The model under review builds one solid part; all positions refer to its coordinate system, in mm. A direction names the side the tool comes from. Coordinates: 2 decimals unless noted, no trailing zeros. Write each loop counter-clockwise with the first axis right and the second up, starting at its lowest first coordinate (ties: lowest second). Pieces come first, ordered by that corner, then holes.
```python
from build123d import *

# Parameters (mm, degrees)
SCHIZZO1_R                                   = 40
ESTRUSIONE_ESTRUSIONE1_DEPTH                 = 45
SCHIZZO2_W                                   = 156
SCHIZZO2_H                                   = 140
SCHIZZO2_R                                   = 30
ESTRUSIONE_ESTRUSIONE2_DEPTH                 = 25
ESTRUSIONE_ESTRUSIONE4_DEPTH                 = 10
SCHIZZO6_R                                   = 12.5
TAGLIO_ESTRUSIONE1_DEPTH                     = 10
FORO_LAMATO_PER_VITE_M4_A_TESTA_ESAG_2_COUNT = 2
FORO_LAMATO_PER_VITE_M4_A_TESTA_ESAG_2_PITCH = 36.062445841
FORO_LAMATO_PER_VITE_M4_A_TESTA_ESAG_3_COUNT = 2
FORO_LAMATO_PER_VITE_M4_A_TESTA_ESAG_3_PITCH = 51
FORO_LAMATO_PER_VITE_M4_A_TESTA_ESAG_4_COUNT = 2
FORO_LAMATO_PER_VITE_M4_A_TESTA_ESAG_4_PITCH = 36.062445841
FORO_PER_VITE_M5_1_D                         = 5.5


with BuildPart() as part:
    # Schizzo1 → Estrusione-Estrusione1 (new body)
    with BuildSketch(Plane(origin=(0, 0, 0), x_dir=(0, 0, -1), z_dir=(1, 0, 0))):
        with BuildLine():
            Line((-70, 0), (-70, 136.8))
            Line((-70, 136.8), (70, 136.8))
            Line((70, 136.8), (70, 0))
            ThreePointArc((70, 0), (0, -70), (-70, 0))
        make_face()
        with Locations(Location((0, 0, 0), (0, 0, 180))):
            Circle(SCHIZZO1_R, mode=Mode.SUBTRACT)
    extrude(amount=ESTRUSIONE_ESTRUSIONE1_DEPTH)

    # Schizzo2 → Estrusione-Estrusione2 (add)
    with BuildSketch(Plane(origin=(0, 136.8, 0), x_dir=(1, 0, 0), z_dir=(0, 1, 0))):
        with Locations((78, 0)):
            Rectangle(SCHIZZO2_W, SCHIZZO2_H)
        with Locations(Location((93.7, 0, 0), (0, 0, 270))):
            Circle(SCHIZZO2_R, mode=Mode.SUBTRACT)
    extrude(amount=ESTRUSIONE_ESTRUSIONE2_DEPTH)

    # Schizzo5 → Estrusione-Estrusione4 (add)
    with BuildSketch(Plane(origin=(0, 161.8, 0), x_dir=(1, 0, 0), z_dir=(0, 1, 0))):
        Polygon((156, 170), (156, 70), (0, 70), (0, -70), (-44, -70), (-44, 170), align=None)
    extrude(amount=-ESTRUSIONE_ESTRUSIONE4_DEPTH)

    # Schizzo6 → Taglio-Estrusione1 (cut)
    with BuildSketch(Plane(origin=(0, 161.8, 0), x_dir=(1, 0, 0), z_dir=(0, 1, 0))):
        with Locations(Location((7.7, 125, 0), (0, 0, 270))):
            Circle(SCHIZZO6_R)
    extrude(amount=-TAGLIO_ESTRUSIONE1_DEPTH, mode=Mode.SUBTRACT)

    # Schizzo8 → Foro lamato per Vite M4 a testa esagonale-1 (revolve, cut)
    with BuildSketch(Plane(origin=(7.7, 161.8, -150.5), x_dir=(0, 0, 1), z_dir=(1, 0, 0))):
        Polygon((0, 0), (0, 231.8), (2.25, 231.8), (2.25, 2.8), (5.5415, 2.8), (5.5415, 0.025), (5.5665, 0), align=None)
    foro_lamato_per_vite_m4_a_testa_esagonal = revolve(axis=Axis((7.7, 168.15, -150.5), (0, -1, 0)), mode=Mode.SUBTRACT)

    # Foro lamato per Vite M4 a testa esag 2: Foro lamato per Vite M4 a testa esagonale-1 ×2
    with Locations(*[Vector(-0.7071067811865476, 0, 0.7071067811865476) * (i * FORO_LAMATO_PER_VITE_M4_A_TESTA_ESAG_2_PITCH) for i in range(1, FORO_LAMATO_PER_VITE_M4_A_TESTA_ESAG_2_COUNT)]):
        add(foro_lamato_per_vite_m4_a_testa_esagonal, mode=Mode.SUBTRACT)

    # Foro lamato per Vite M4 a testa esag 3: Foro lamato per Vite M4 a testa esagonale-1 ×2
    with Locations(*[(0, 0, i * FORO_LAMATO_PER_VITE_M4_A_TESTA_ESAG_3_PITCH) for i in range(1, FORO_LAMATO_PER_VITE_M4_A_TESTA_ESAG_3_COUNT)]):
        add(foro_lamato_per_vite_m4_a_testa_esagonal, mode=Mode.SUBTRACT)

    # Foro lamato per Vite M4 a testa esag 4: Foro lamato per Vite M4 a testa esagonale-1 ×2
    with Locations(*[Vector(0.7071067811865475, 0, 0.7071067811865476) * (i * FORO_LAMATO_PER_VITE_M4_A_TESTA_ESAG_4_PITCH) for i in range(1, FORO_LAMATO_PER_VITE_M4_A_TESTA_ESAG_4_COUNT)]):
        add(foro_lamato_per_vite_m4_a_testa_esagonal, mode=Mode.SUBTRACT)

    # Foro per Vite M5-1 (through all)
    with Locations(Plane(origin=(0, 161.8, 0), x_dir=(1, 0, 0), z_dir=(0, 1, 0))):
        with Locations((93.7, 38), (93.7, -38), (55.7, 0), (131.7, 0)):
            Hole(FORO_PER_VITE_M5_1_D / 2)


solid = part.part
```
Item 1: Machinability: for faces 1 (the face through (41, 99, 70)), 2 (the face through (10.1, 159, -150.4)), 3 (the face through (42, 92, -70)), which of the approach directions +Z, -Z, +X, -X, +Y, -Y give a long, thin tool a straight path to every point of the face, cutting with its end or side? Answer none if there is none.
Solved:
face 1: +Z, +X, -X, +Y, -Y
face 2: +Y
face 3: -Z, +X, -X, -Y
Item 2: Take a section at C-C, the plane y = 22. Write out the cut boundary in (x, z), plus the area to 3 significant figures.
Solved:
outline: (0, -70) - (45, -70) - (45, -33.41) - (0, -33.41) - close; (0, 33.41) - (45, 33.41) - (45, 70) - (0, 70) - close
area: 3,290 mm2
Item 3: Take a section at D-D, the plane y = 63.5. Write out the cut boundary in (x, z).
Solved:
outline: (0, -70) - (45, -70) - (45, 70) - (0, 70) - close
Item 4: For pin 1 (3 mm diameter, centred on x = 13, z = -117.5, fed in from -Y) (3 decimals); pin 2 (3 mm diameter, centred on x = 23, y = -9.5, fed in from -Z); pin 3 (5 mm diameter, centred on x = 7.7, z = -99.5, fed in from +Y); pin 4 (1.5 mm diameter, centred on x = 16, y = 103.5, fed in from -Z), all flat-tipped, find the tip position at first contact; note any pin that passes through.
Solved:
pin 1: passes through
pin 2: stops at z = -69.54
pin 3: stops at y = 159
pin 4: stops at z = -70
Item 5: Take a section at A-A, the plane y = -12.5. Write out the cut boundary in (x, z).
Solved:
outline: (0, -68.87) - (45, -68.87) - (45, -38) - (0, -38) - close; (0, 38) - (45, 38) - (45, 68.87) - (0, 68.87) - close
Item 6: Mouldability with a two-part tool opening along X and no side actions: class faces 4 (the face through (36, 159, -125)), 5 (the face through (0, 64, 1)), 6 (the face through (124, 136.8, -1)) as pulls with the +X half, pulls with the -X half, needs draft (parallel to the pull), parting line crosses it, or undercut.
Solved:
face 4: undercut
face 5: pulls with the -X half
face 6: needs draft
Item 7: To check wall thickness, follow line 1 along X through (y, z) = (159.85, -125); line 2 along Z through (x, y) = (33, 157); line 3 along X through (y, z) = (153, -150). State the ranges of each line that lie inside material, in increasing order.
Solved:
line 1: x = -44 to -23.34, -12.26 to -4.8, 20.2 to 27.66, 38.74 to 156
line 2: z = -170 to -127.24, -122.76 to 70
line 3: x = -44 to 5.51, 9.89 to 156
Item 8: Take a section at B-B, the plane z = -61. Write out the cut boundary in (x, y), plus the area to 3 significant figures.
Solved:
outline: (-44, 151.8) - (0, 151.8) - (0, -34.34) - (45, -34.34) - (45, 136.8) - (156, 136.8) - (156, 161.8) - (-44, 161.8) - close
area: 12,000 mm2
